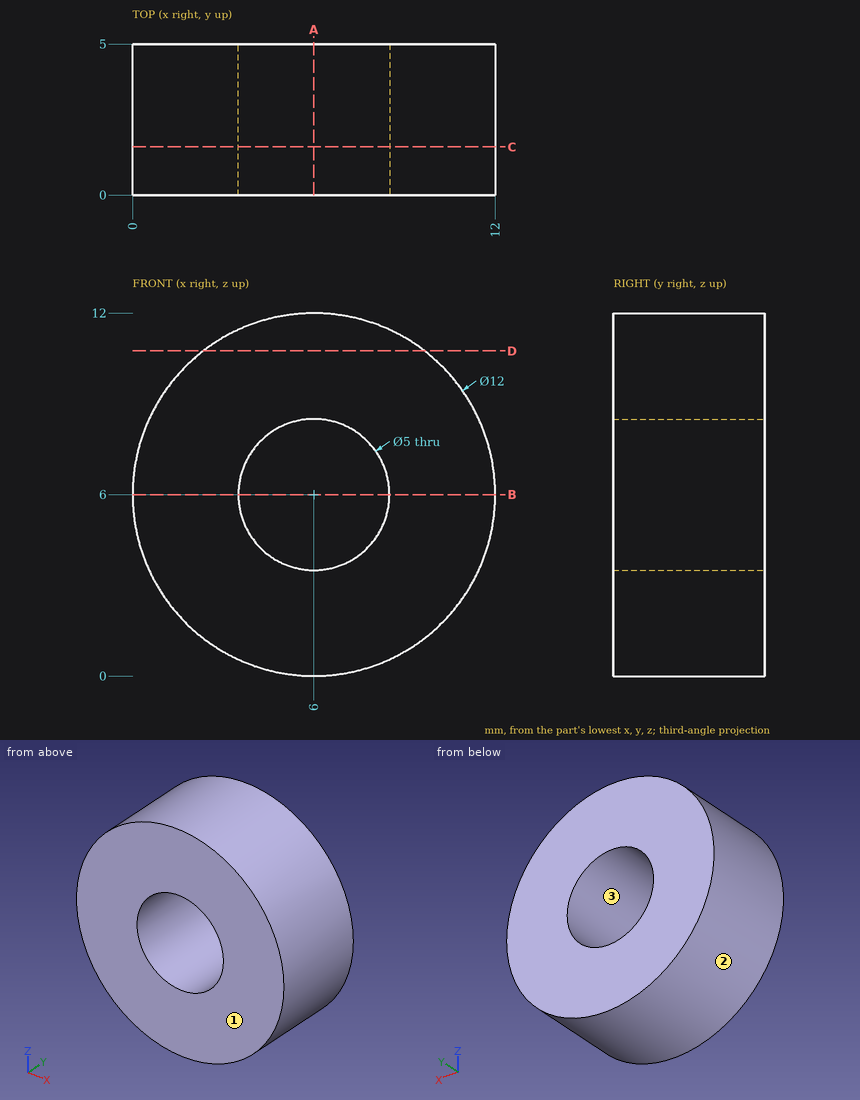
The figure shows three views and two pictorial views of one solid part (mm, origin at its lowest corner). Answer the questions. Coordinates: 2 decimals unless noted, no trailing zeros. Write each loop counter-clockwise with the first axis right and the second up, starting at its lowest first coordinate (ties: lowest second). Pieces come first, ordered by that corner, then holes. Notation, with made-up numbers: (76, -2.75) -> (106, -2.75) arc R13 ccw to (106, 15.25) -> close; hole circle Ø9 at (-12.75, 33.25). An arc over 180 degrees is marked (long way). Return JSON: item names as keys, results as strings.
(1) The part is cut by section B-B on z = 6. Give the vertices of the cut face in (x, y).
Answers below:
{"outline": "(0, 0) -> (3.5, 0) -> (3.5, 5) -> (0, 5) -> close; (8.5, 0) -> (12, 0) -> (12, 5) -> (8.5, 5) -> close"}
(2) This flat-tipped pin is pushed along its axis until it touches: P1, Ø1.5, axis at x = 8.5, z = 8.5, coming from the -Y side. Where does it stop, or does it pass through?
Answers below:
{"P1": "y = 0"}
(3) The part is cut by section D-D on z = 10.75. Give the vertices of the cut face in (x, y).
Answers below:
{"outline": "(2.33, 0) -> (9.67, 0) -> (9.67, 5) -> (2.33, 5) -> close"}
(4) The part is cut by section A-A on x = 6. Give the vertices of the cut face in (y, z), then the cut area to 3 significant figures.
Answers below:
{"outline": "(0, 0) -> (5, 0) -> (5, 3.5) -> (0, 3.5) -> close; (0, 8.5) -> (5, 8.5) -> (5, 12) -> (0, 12) -> close", "area": "35.0 mm^2"}
(5) The part is cut by section C-C on y = 1.6. Give the vertices of the cut face in (x, z), then the cut area to 3 significant figures.
Answers below:
{"outline": "circle Ø12 at (6, 6); hole circle Ø5 at (6, 6)", "area": "93.5 mm^2"}
(6) For a pull along X with two mould halves and no side action, classify the marked faces 1, 2 and 3 as pulls with the +X half, pulls with the -X half, needs draft (parallel to the pull), parting line crosses it, or undercut.
Answers below:
{"face 1": "needs draft", "face 2": "parting line crosses it", "face 3": "undercut"}
(7) Consider line 1 along Z through (x, y) = (6, 2.4); line 2 along X through (y, z) = (4.3, 4.25). Determine where each line is inside the solid, lowest interval first. Write a range as from..to.
Answers below:
{"line 1": "0..3.5, 8.5..12", "line 2": "0.26..4.21, 7.79..11.74"}
